Job drawing, mm, ordinate dimensions from the low corner. One solid piece. A direction names the side the tool comes from. Give positions to 0.01 mm unless a question says otherwise; leave off trailing zeros. Write each loop counter-clockwise with the first axis right and the second up, starting at its lowest first coordinate (ties: lowest second). Pieces come first, ordered by that corner, then holes. Notation, with made-up numbers: M -9.5,44 L 29.5,44 A28 ccw 29.5,73 Z; hole C -18,49 d3. An arc over 180 degrees is marked long. Answer as CSV lines item,"result". Start each with the question number.
1) Pin check, flat tips, straight feed: pin 1 Ø6 at (x, z) = (46.5, 6.5) entering from +Y (1 decimal); pin 2 Ø1 at (x, z) = (41, 13) entering from +Y; pin 3 Ø6 at (x, z) = (30, 5.5) entering from +Y. Stop position of each tip, or through.
2) Mould opens along X. For the marked faces 1, 2 and 3 say: pulls with the +X half, pulls with the -X half, needs draft (parallel to the pull), parting line crosses it, or undercut.
3) Tool access for the marked faces 4 and 5: list every direction of +Z, -Z, +X, -X, +Y, -Y with a clear straight run to the whole face (end or side of a thin tool).
4) Wall check: line 1 along X through (y, z) = (57, 17.5); line 2 along Y through (x, z) = (10.5, 16.5); line 3 along Y through (x, z) = (53.5, 11.25). Give the ranges that are in metal, low to high. Write a range as from..to.
5) Slice it at A-A, the plane y = 30. Give the cut face in (x, z).
6) Slice it at D-D, the plane z = 12.75. Give the cut face in (x, y) (1 decimal), plus the area to 3 significant figures.
7) Slice it at C-C, the plane y = 45. Give the cut face in (x, z).
8) Slice it at B-B, the plane x = 20. Give the cut face in (y, z).
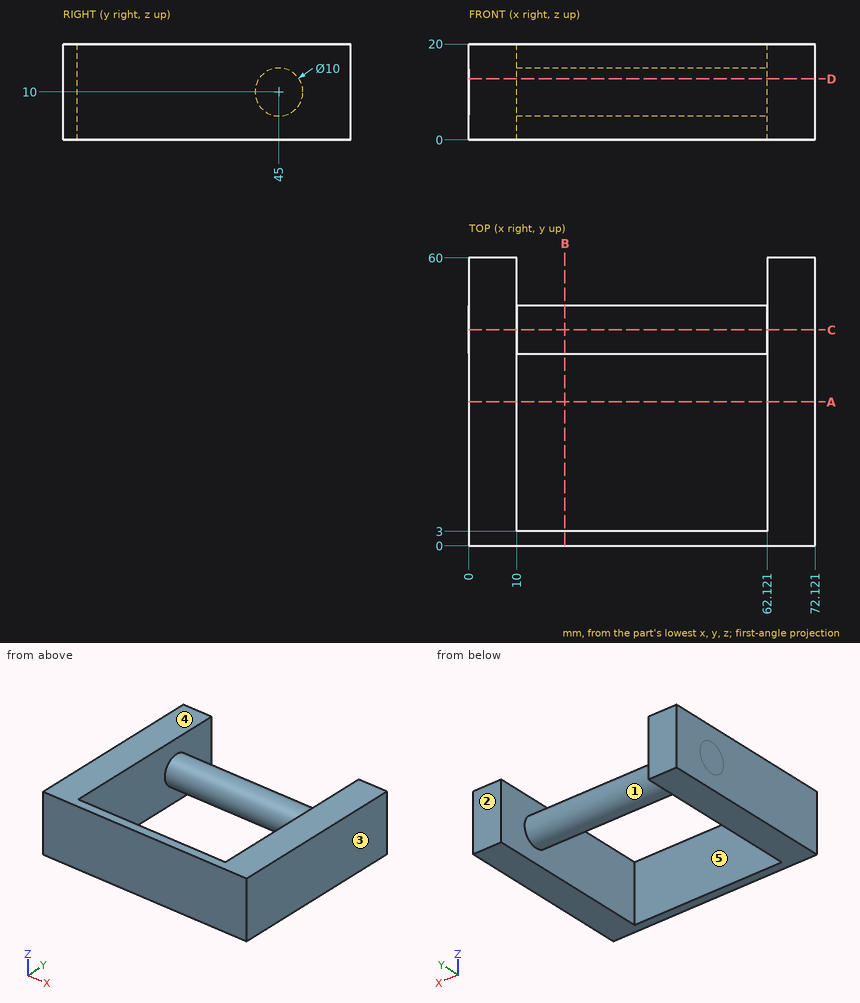
Found:
1,pin 1,"y = 50"
1,pin 2,"y = 49.33"
1,pin 3,"y = 49.77"
2,face 1,"undercut"
2,face 2,"needs draft"
2,face 3,"pulls with the +X half"
3,face 4,"+Z, +X, -X, +Y, -Y"
3,face 5,"+Z, -Z"
4,line 1,"0..10, 62.12..72.12"
4,line 2,"0..3"
4,line 3,"0..3, 40.16..49.84"
5,outline,"M 0,0 L 10,0 L 10,20 L 0,20 Z; M 62.12,0 L 72.12,0 L 72.12,20 L 62.12,20 Z"
6,outline,"M 0,0 L 72.1,0 L 72.1,60 L 62.1,60 L 62.1,49.2 L 10,49.2 L 10,60 L 0,60 Z; hole M 10,3 L 62.1,3 L 62.1,40.8 L 10,40.8 Z"
6,area,"1,790 mm²"
7,outline,"M 0,0 L 10,0 L 10,5 L 62.12,5 L 62.12,0 L 72.12,0 L 72.12,20 L 62.12,20 L 62.12,15 L 10,15 L 10,20 L 0,20 Z"
8,outline,"M 0,0 L 3,0 L 3,20 L 0,20 Z; C 45,10 d10"
